Answer from the drawing. Dimensions are ordinates in mm from the lowest x, y and z of the part. A direction names the side the tool comes from. Round coordinates to 2 decimals unless told otherwise and drop trailing zeros. Order: outer loops, then holes, each group sorted by start corner. A loop starts at its lowest first (then second) coordinate and runs counter-clockwise, first axis right, second up. Notation, with made-up numbers: (-11.5, -23.75) - (-2.5, -23.75) arc R26 cw to (-2.5, 4.25) - close; hole circle Ø7 at (59, 41.25). An arc over 180 degrees is marked (long way). One line per question, with ' | ' between items. Start each with the question number.
1) For the marked faces 1 and 2, determine the directions among +Z, -Z, +X, -X, +Y, -Y from which every point of the face is accessible in a straight line to the end or side of a thin tool.
2) The mould has two halves that part along Y. Classify the marked faces 3, 4 and 5: pulls with the +Y half, pulls with the -Y half, needs draft (parallel to the pull), parting line crosses it, or undercut.
3) The part is cut by section B-B, the plane x = 10. Give the vertices of the cut face in (y, z), plus the area to 3 significant figures.
4) The part is cut by section C-C, the plane y = 10. Give the vertices of the cut face in (x, z).
5) The part is cut by section A-A, the plane z = 20. Give the vertices of the cut face in (x, y), plus the area to 3 significant figures.
6) The part is cut by section D-D, the plane z = 2.75. Give the vertices of the cut face in (x, y).
7) Flat-ended cylindrical pins translate along their axes: pin 1 (8 mm diameter, centred on x = 23.5, y = 17.5, fed in from +Z); pin 2 (3 mm diameter, centred on x = 25, z = 20, fed in from -Y); pin 3 (6 mm diameter, centred on x = 23.5, y = 14, fed in from +Z). Find the tip coordinate at first contact, or state that the pin passes through.
8) Straight lines are drawn through the part: line 1 (Y direction, x = 10, z = 7.5); line 2 (Z direction, x = 10, y = 26.75); line 3 (X direction, y = 28.5, z = 21.75). For each, find the intervals that lie inside material, in ascending order. Write a range as from..to.
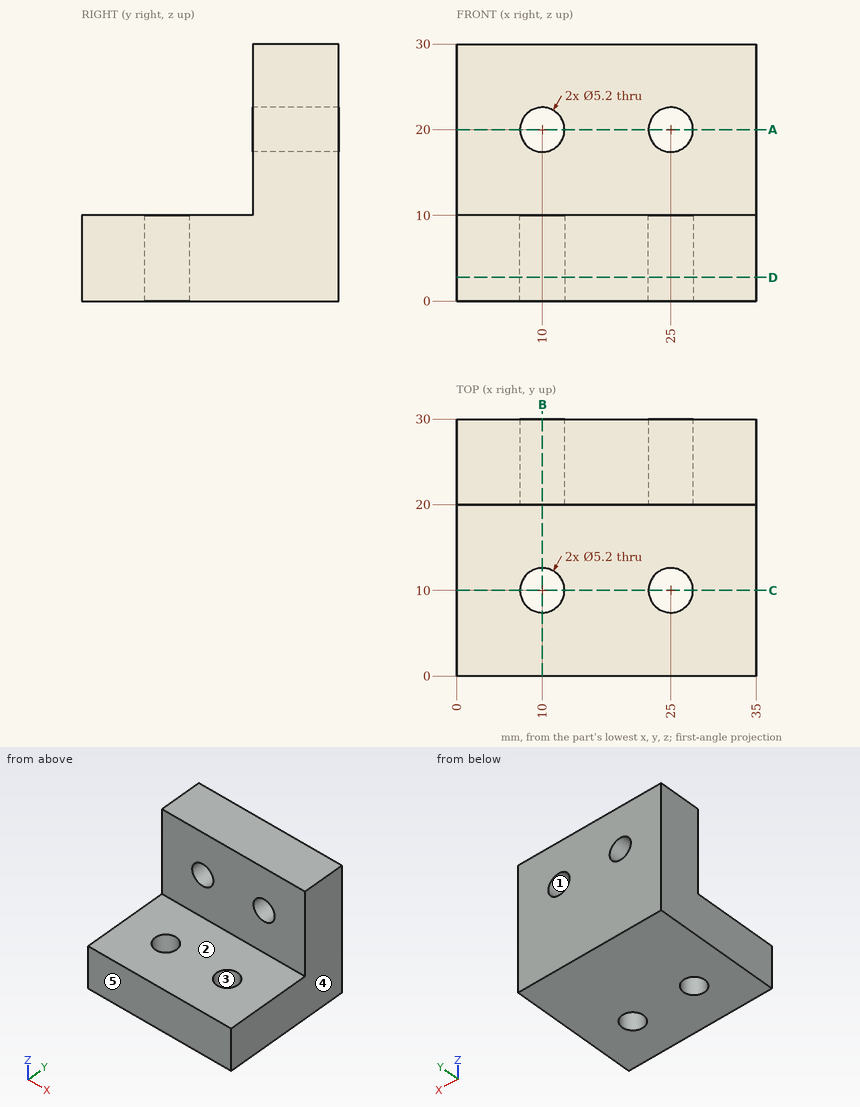
Values:
1) face 1: +Y, -Y | face 2: +Z, +X, -X, -Y
2) face 3: undercut | face 4: needs draft | face 5: pulls with the -Y half
3) outline: (0, 0) - (7.4, 0) - (7.4, 10) - (0, 10) - close; (12.6, 0) - (30, 0) - (30, 17.4) - (20, 17.4) - (20, 10) - (12.6, 10) - close; (20, 22.6) - (30, 22.6) - (30, 30) - (20, 30) - close | area: 396 mm^2
4) outline: (0, 0) - (7.4, 0) - (7.4, 10) - (0, 10) - close; (12.6, 0) - (22.4, 0) - (22.4, 10) - (12.6, 10) - close; (27.6, 0) - (35, 0) - (35, 10) - (27.6, 10) - close
5) outline: (0, 20) - (7.4, 20) - (7.4, 30) - (0, 30) - close; (12.6, 20) - (22.4, 20) - (22.4, 30) - (12.6, 30) - close; (27.6, 20) - (35, 20) - (35, 30) - (27.6, 30) - close | area: 246 mm^2
6) outline: (0, 0) - (35, 0) - (35, 30) - (0, 30) - close; hole circle Ø5.2 at (10, 10); hole circle Ø5.2 at (25, 10)
7) pin 1: stops at z = 30 | pin 2: passes through | pin 3: stops at z = 10
8) line 1: y = 0..7.4, 12.6..30 | line 2: z = 0..17.4, 22.6..30 | line 3: x = 0..8.08, 11.92..23.08, 26.92..35
